The model under review builds one solid part; all positions refer to its coordinate system, in mm. Face numbers are marked on the shaded views. Coordinates: 2 decimals unless noted, no trailing zeros. Order: outer loops, then holes, each group sorted by start corner. A loop starts at its lowest first (then second) coordinate and runs counter-clockwise, first axis right, second up. Notation, with made-up numbers: (-23.75, -22.5) - (30.25, -22.5) arc R26 ccw to (30.25, 11.5) - close; hole circle Ø10 at (11, 68). An arc over 180 degrees is marked (long way). Answer in a Markdown table with one row per item.
```python
from build123d import *

# Parameters (mm, degrees)
F0_R     = 22.225
F1_DEPTH = 3.175
F2_R     = 12.7
F3_DEPTH = 44.45
F4_R     = 22.225
F5_DEPTH = 3.175
F6_R     = 0.635
F7_DEPTH = 50.8
F8_T     = -1.778


# Not quite as in the source:
# - a length typed as a fraction of an inch, garbled in the dataset ("3 / 203.2 mm" for 3/8 in), is restored


with BuildPart() as f1:
    # F0 (on Top) → F1 (new body)
    with BuildSketch(Plane.XY):
        Circle(F0_R)
    extrude(amount=F1_DEPTH)

    # F2 (on face) → F3 (join)
    with BuildSketch(Plane(origin=(0, 0, 0), x_dir=(1, 0, 0), z_dir=(0, 0, -1))):
        Circle(F2_R)
    extrude(amount=F3_DEPTH)

    # F4 (on face) → F5 (join)
    with BuildSketch(Plane(origin=(0, 0, -44.45), x_dir=(1, 0, 0), z_dir=(0, 0, -1))):
        Circle(F4_R)
    extrude(amount=F5_DEPTH)

    # F6 (on face) → F7 (cut, through all)
    with BuildSketch(Plane.XY.offset(3.175)):
        with BuildLine():
            ThreePointArc((-3.175, 0), (0, -3.175), (3.175, 0))
            ThreePointArc((3.175, 0), (0, 3.175), (-3.175, 0))
        make_face()
        with BuildLine():
            ThreePointArc((-17.145, 0), (-16.51, -0.635), (-15.875, 0))
            Line((-15.875, 0), (-17.145, 0))
        make_face()
        with BuildLine():
            Line((-17.145, 0), (-15.875, 0))
            ThreePointArc((-15.875, 0), (-16.51, 0.635), (-17.145, 0))
        make_face()
        with Locations((16.51, 0)):
            Circle(F6_R)
    extrude(amount=-F7_DEPTH, mode=Mode.SUBTRACT)

    # F8 (hollow: no face is removed)
    offset(amount=F8_T, kind=Kind.INTERSECTION, mode=Mode.SUBTRACT)


solid = f1.part
```
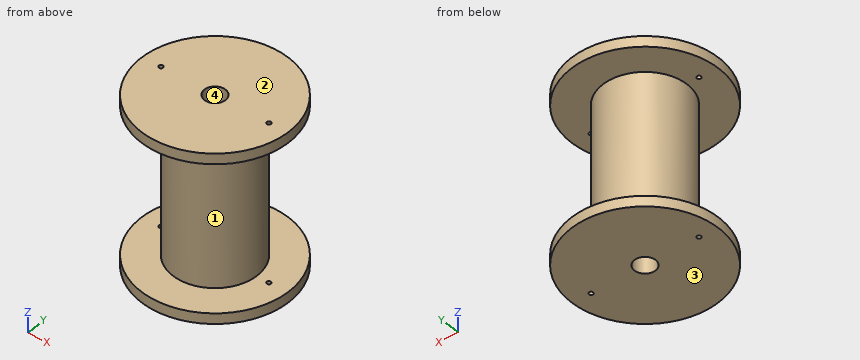
Item 1: We need section A-A, the plane x = 2.5. State how many separate pieces and enclosed holes the cut face has, then the cut area to 3 significant figures.
Check values:
| item | result |
|---|---|
| separate pieces | 2 |
| enclosed holes | 2 |
| area | 588 mm^2 |
Item 2: We need section B-B, the plane z = -39. Write out the cut boundary in (x, y) (3 decimals).
Check values:
| item | result |
|---|---|
| outline | circle Ø25.4 at (0, 0); circle Ø9.906 at (0, 0); hole circle Ø21.844 at (0, 0); hole circle Ø6.35 at (0, 0) |
Item 3: To check wall thickness, follow line 1 (Y direction, x = 0, z = -12) (3 decimals); line 2 (Z direction, x = 16, y = -4) (3 decimals); line 3 (Z direction, x = 7, y = -2.5) (3 decimals). State the ranges of each line that lie inside material, in increasing order. Write a range as from..to.
Check values:
| item | result |
|---|---|
| line 1 | -12.7..-10.922, -4.953..-3.175, 3.175..4.953, 10.922..12.7 |
| line 2 | -47.625..-44.45, 0..3.175 |
| line 3 | -47.625..-45.847, 1.397..3.175 |
Item 4: Mouldability with a two-part tool opening along Z and no side actions: class the marked faces 1, 2, 3 and 4 as +Z half, -Z half, draft (parallel to the pull), parting line (faces both ways), or undercut.
Check values:
| item | result |
|---|---|
| face 1 | undercut |
| face 2 | +Z half |
| face 3 | -Z half |
| face 4 | draft |
Item 5: We need section C-C, the plane y = -18.5. Write out the cut boundary in (x, z) (3 decimals), then the cut area to 3 significant figures.
Check values:
| item | result |
|---|---|
| outline | (-12.317, -47.625) - (12.317, -47.625) - (12.317, -44.45) - (-12.317, -44.45) - close; (-12.317, 0) - (12.317, 0) - (12.317, 3.175) - (-12.317, 3.175) - close |
| area | 156 mm^2 |
Item 6: Clearance check with flat-ended pins moving along their axes: pin 1 Ø6 at (x, z) = (-4.5, -40.5) entering from -Y; pin 2 Ø6 at (y, z) = (7, -9) entering from -X; pin 3 Ø12 at (x, z) = (9, -2) entering from -Y. State where each tip first meets the part, or that it passes through.
Check values:
| item | result |
|---|---|
| pin 1 | y = -12.61 |
| pin 2 | x = -12.05 |
| pin 3 | y = -21.97 |
